Could you check a few things on this model? Use its own coordinates, in mm. A direction names the side the tool comes from. Coordinates: 2 decimals unless noted, no trailing zeros. Loops run counter-clockwise (first coordinate to the right, second up) from the corner with the lowest first, then second, coordinate; pieces in that order, holes last.
from build123d import *

# Parameters (mm, degrees)
F0_W     = 101.6
F0_H     = 50.8
F0_R     = 15.875
F1_DEPTH = 25.4
F2_W     = 6.35
F2_H     = 50.8
F3_DEPTH = 2.54
F5_DEPTH = 50.801
F6_R     = 4.7625
F7_DEPTH = 12.7
F8_R     = 25.4
F8_R_2   = 4.7625
F9_DEPTH = 6.35


with BuildPart() as f1:
    # F0 (on Top) → F1 (new body)
    with BuildSketch(Plane.XY):
        Rectangle(F0_W, F0_H)
        Circle(F0_R, mode=Mode.SUBTRACT)
    extrude(amount=F1_DEPTH)

    # F2 (on face) → F3 (cut)
    with BuildSketch(Plane.XY.offset(25.4)):
        with BuildLine():
            Line((6.35, 25.4), (-6.35, 25.4))
            Line((-6.35, 25.4), (-6.35, 14.5496778315))
            ThreePointArc((-6.35, 14.5496778315), (0, 15.875), (6.35, 14.5496778315))
            Line((6.35, 14.5496778315), (6.35, 25.4))
        make_face()
        with BuildLine():
            Line((-6.35, -14.5496778315), (-6.35, -25.4))
            Line((-6.35, -25.4), (6.35, -25.4))
            Line((6.35, -25.4), (6.35, -14.5496778315))
            ThreePointArc((6.35, -14.5496778315), (0, -15.875), (-6.35, -14.5496778315))
        make_face()
        with Locations((-45.085, 0)):
            Rectangle(F2_W, F2_H)
    extrude(amount=-F3_DEPTH, mode=Mode.SUBTRACT)

    # F4 (on face) → F5 (cut, through all)
    with BuildSketch(Plane.XZ.offset(25.4)):
        Polygon((31.75, 25.4), (19.05, 25.4), (16.1170606325, 20.32), (34.6829393675, 20.32), align=None)
    extrude(amount=-F5_DEPTH, mode=Mode.SUBTRACT)

    # F6 (on face) → F7 (join)
    with BuildSketch(Plane.YZ.offset(50.8)):
        with Locations((0, 12.7)):
            Circle(F6_R)
    extrude(amount=F7_DEPTH)

    # F8 (on face) → F9 (join)
    with BuildSketch(Plane.YZ.offset(63.5)):
        with Locations((0, 12.7)):
            Circle(F8_R)
        with Locations((0, 12.7)):
            Circle(F8_R_2, mode=Mode.SUBTRACT)
        with Locations((0, 12.7)):
            Circle(F8_R_2)
    extrude(amount=F9_DEPTH)


solid = f1.part
1) Imagine slicing it at B-B on x = 0. List the corners of the cut face in (y, z) for me (3 decimals).
2) Imagine slicing it at D-D on y = 6.5. List the corners of the cut face in (x, z) for me, plus the area to 3 significant figures.
3) We'd pull the mould along X, two halves only. Please class faces 6 (the flat face through (69.85, 0, 13)), 7 (the flat face through (6.35, 20, 24)), 8 (the flat face through (-1, 25.4, 13)), 9 (the flat face through (-6.35, -20, 24)): released by +X, released by -X, zero draft, split by the parting line, or undercut.
4) For faces 1 (the flat face through (-1, -25.4, 13)), 2 (the flat face through (17.604, -0.356, 22.896)), 3 (the flat face through (-24, 0, 25.4)), 4 (the cylindrical face through (57.06, -1.03, 8.05)), 5 (the flat face through (-41.91, 0, 24)), which set-ups out of +Z, -Z, +X, -X, +Y, -Y let a thin tool reach every point of the face, with its end or its side?
5) Will these pins go through, and if not, where does the flat tip stop? pin 1 (12 mm diameter, centred on x = -1.5, y = 17.5, fed in from +Z); pin 2 (10 mm diameter, centred on x = 30.5, y = -15.5, fed in from -Z); pin 3 (19 mm diameter, centred on x = 0, y = 0, fed in from +Z).
6) If I drill on L1, parallel to X at y = 0, z = 5.75 (3 decimals); L2, parallel to X at y = -11.5, z = 18; L3, parallel to Y at x = 0, z = 11 (3 decimals), over which ranges is the centre line in solid material (lowest first)?
Solved:
1. outline: (-25.4, 0) - (-15.875, 0) - (-15.875, 22.86) - (-25.4, 22.86) - close; (15.875, 0) - (25.4, 0) - (25.4, 22.86) - (15.875, 22.86) - close
2. outline: (-50.8, 0) - (-14.48, 0) - (-14.48, 25.4) - (-41.91, 25.4) - (-41.91, 22.86) - (-48.26, 22.86) - (-48.26, 25.4) - (-50.8, 25.4) - close; (14.48, 0) - (50.8, 0) - (50.8, 25.4) - (31.75, 25.4) - (34.68, 20.32) - (16.12, 20.32) - (19.05, 25.4) - (14.48, 25.4) - close; (63.5, -11.85) - (69.85, -11.85) - (69.85, 37.25) - (63.5, 37.25) - close
2. area: 2,060 mm2
3. face 6: released by +X
3. face 7: undercut
3. face 8: zero draft
3. face 9: undercut
4. face 1: +Z, -Z, +X, -X, -Y
4. face 2: +Y, -Y
4. face 3: +Z, -X, +Y, -Y
4. face 4: none
4. face 5: +Z, +Y, -Y
5. pin 1: stops at z = 25.4
5. pin 2: stops at z = 0
5. pin 3: passes through
6. L1: x = -50.8 to -15.875, 15.875 to 50.8, 63.5 to 69.85
6. L2: x = -50.8 to -10.94, 10.94 to 50.8, 63.5 to 69.85
6. L3: y = -25.4 to -15.875, 15.875 to 25.4
